Check sheet for the modelled part. Datum: model origin and axes. Units: mm. A direction names the side the tool comes from. Give positions to 0.01 mm unless a question says otherwise; leave off trailing zeros. Write each loop counter-clockwise with the first axis right and the second up, starting at its lowest first coordinate (ties: lowest second). Pieces come first, ordered by that corner, then holes. Notation, with made-up numbers: M -11.75,-11 L 30.25,-11 A28 ccw 30.25,26 Z; hole C 56,81 d3. An arc over 180 degrees is marked long. Use CSV: the item, a comma, the result in double quotes. Start each with the question number.
1. Cross-section at A-A, the plane z = 9. Enter the section's corners in (x, y), and give its area (3 significant figures).
2. Mould release check, pull along X, two halves, no side actions. Record for faces 1 (the face through (-2.37, 35.92, 4.93)), 2 (the face through (29.97, 1.32, 5.94)), 3 (the face through (14, -27, 10)): +X half, -X half, draft (parallel to the pull), parting line (faces both ways), or undercut.
3. Access from +Z, -Z, +X, -X, +Y, -Y to the whole of each face (thin tool, end or side, straight path). Record for faces 4 (the face through (6.2, -6.2, 2)), 5 (the face through (-4, 0, 10)).
4. Depth check by flat-ended pin: P1, Ø2, axis at x = -15.5, z = 7.5, coming from the +Y side; P2, Ø5, axis at x = -21.5, z = 3, coming from the +Y side; P3, Ø18, axis at x = 7.5, y = -12, coming from the +Z side; P4, Ø3.5, axis at x = 0, y = 0, coming from the -Z side. Enter the tip coordinate at first touch or a pass-through.
5. Scan lines: line 1 (Y direction, x = 0, z = 5.25); line 2 (X direction, y = 4.5, z = 4.25). Record each from-to range of solid material in increasing order.
6. Cross-section at C-C, the plane y = -12.5. Enter the section's corners in (x, z), and give its area (3 significant figures).
Autodesk Fusion 360 part; units mm, degrees
sketch "Sketch1" plane through (0, 0, 0) normal (0, 0, 1) x (1, 0, 0)
  circle A0 centre (0, 0) radius 36
  circle A1 centre (0, 0) radius 3
  dimension "d1" = 72
  dimension "d2" = 6
extrude "Extrude1" add sketch "Sketch1" along normal blind 2
sketch "Sketch2" plane through (0, 0, 2) normal (0, 0, 1) x (-1, 0, 0)
  circle A0 centre (0, 0) radius 3
  circle A1 centre (0, 0) radius 36
  circle A2 centre (0, 0) radius 30
  circle A3 centre (0, 0) radius 8.5
  dimension "d5" = 60
  dimension "d6" = 17
extrude "Extrude2" add sketch "Sketch2" along normal blind 8
Worked answers:
1,outline,"C 0,0 d72; C 0,0 d17; hole C 0,0 d60; hole C 0,0 d6"
1,area,"1,440 mm^2"
2,face 1,"parting line"
2,face 2,"undercut"
2,face 3,"draft"
3,face 4,"+Z"
3,face 5,"+Z, +X, -X, +Y, -Y"
4,P1,"stops at y = 32.95"
4,P2,"stops at y = 30.58"
4,P3,"stops at z = 10"
4,P4,"passes through"
5,line 1,"y = -36 to -30, -8.5 to -3, 3 to 8.5, 30 to 36"
5,line 2,"x = -35.72 to -29.66, -7.21 to 7.21, 29.66 to 35.72"
6,outline,"M -33.76,0 L 33.76,0 L 33.76,10 L 27.27,10 L 27.27,2 L -27.27,2 L -27.27,10 L -33.76,10 Z"
6,area,"239 mm^2"
